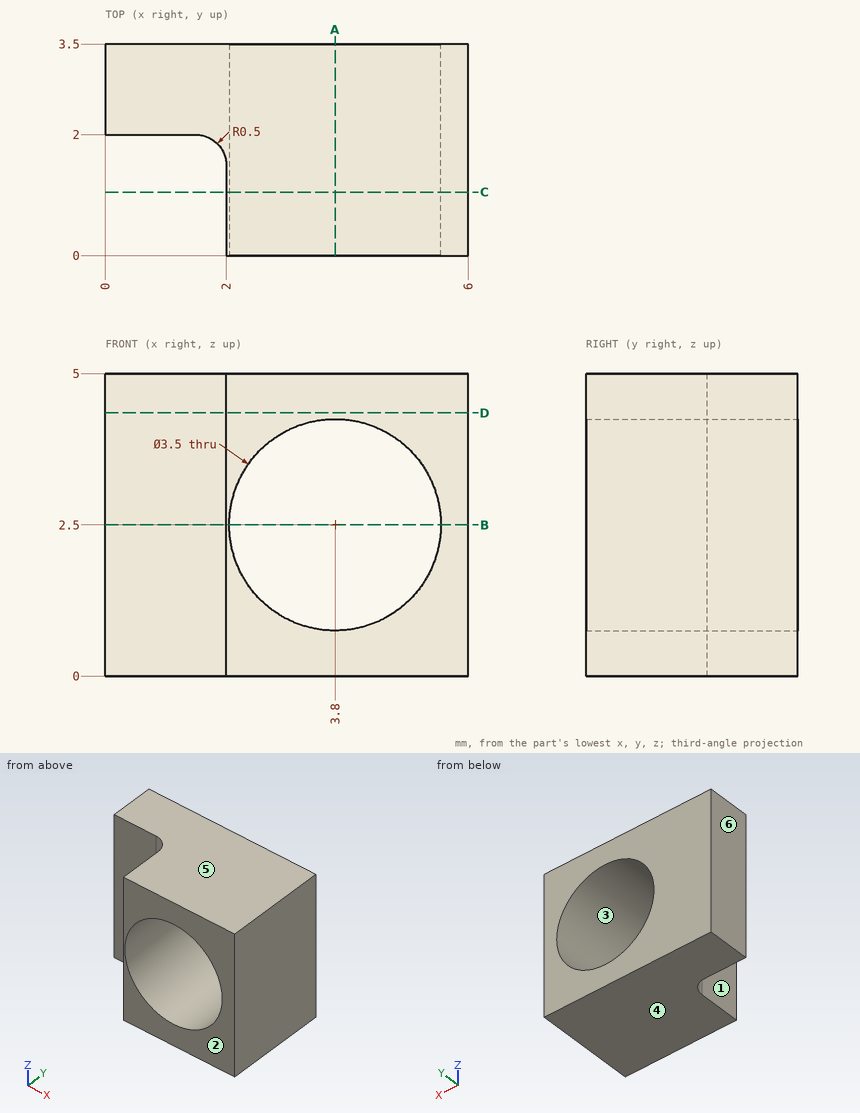
Here's the drawing with two shaded views (mm, measured from the low corner). I have some questions. A direction names the side the tool comes from. Round coordinates to 2 decimals unless told otherwise and drop trailing zeros. Loops run counter-clockwise (first coordinate to the right, second up) from the corner with the lowest first, then second, coordinate; pieces in that order, holes last. Notation, with made-up numbers: M 53,-4.75 L 92,-4.75 A20 cw 92,30.25 Z; hole C 76,36 d9. An arc over 180 degrees is marked long. Answer as CSV lines item,"result".
1) For pin 1 Ø2 at (x, z) = (3.8, 2.5) entering from +Y; pin 2 Ø1.2 at (x, z) = (1, 1.5) entering from -Y, each with a flat end and sliding along its axis, tell me the tip position at first contact or that it passes through.
From the geometry:
pin 1,"through"
pin 2,"y = 1.99"
2) Which directions (+Z, -Z, +X, -X, +Y, -Y) give clear straight access to the entire face, cutting with the end or side of a thin tool? Please do the marked faces 1 and 2.
From the geometry:
face 1,"+Z, -Z, -X, -Y"
face 2,"+Z, -Z, +X, -X, -Y"
3) Imagine slicing it at C-C on y = 1.05. List the corners of the cut face in (x, z) for me, and give its area (3 significant figures).
From the geometry:
outline,"M 2,0 L 6,0 L 6,5 L 2,5 Z; hole C 3.8,2.5 d3.5"
area,"10.4 mm^2"
4) If I drill on probe 1 along Z at (x, y) = (3.8, 1.55); probe 2 along Y at (x, z) = (1.2, 2.1); probe 3 along Z at (x, y) = (3, 2.7), over which ranges is the centre line in solid material (lowest first)?
From the geometry:
probe 1,"0 to 0.75, 4.25 to 5"
probe 2,"2 to 3.5"
probe 3,"0 to 0.94, 4.06 to 5"
5) Imagine slicing it at D-D on z = 4.35. List the corners of the cut face in (x, y) for me, and give its area (3 significant figures).
From the geometry:
outline,"M 0,2 L 1.5,2 A0.5 cw 2,1.5 L 2,0 L 6,0 L 6,3.5 L 0,3.5 Z"
area,"17.1 mm^2"
6) We'd pull the mould along Z, two halves only. Please class the marked faces 3, 4, 5 and 6: released by +Z, released by -Z, zero draft, split by the parting line, or undercut.
From the geometry:
face 3,"undercut"
face 4,"released by -Z"
face 5,"released by +Z"
face 6,"zero draft"
7) Imagine slicing it at B-B on z = 2.5. List the corners of the cut face in (x, y) for me.
From the geometry:
outline,"M 0,2 L 1.5,2 A0.5 cw 2,1.5 L 2,0 L 2.05,0 L 2.05,3.5 L 0,3.5 Z; M 5.55,0 L 6,0 L 6,3.5 L 5.55,3.5 Z"
8) Imagine slicing it at A-A on x = 3.8. List the corners of the cut face in (y, z) for me.
From the geometry:
outline,"M 0,0 L 3.5,0 L 3.5,0.75 L 0,0.75 Z; M 0,4.25 L 3.5,4.25 L 3.5,5 L 0,5 Z"
